from build123d import *

# Parameters (mm, degrees)
SKETCH1_W               = 12.7
SKETCH1_H               = 19.05
BOSS_EXTRUDE1_DEPTH     = 152.4
SKETCH2_R               = 4.5640625
CUT_EXTRUDE1_DEPTH      = 1
CUT_EXTRUDE1_DEPTH_BACK = 13.7
SKETCH6_R               = 2.778125
CUT_EXTRUDE4_DEPTH      = 1
CUT_EXTRUDE4_DEPTH_BACK = 20.05


with BuildPart() as part:
    # Sketch1 → Boss-Extrude1 (new body, symmetric)
    with BuildSketch(Plane(origin=(0, 0, 0), x_dir=(0, 0, -1), z_dir=(1, 0, 0))):
        Rectangle(SKETCH1_W, SKETCH1_H)
    extrude(amount=BOSS_EXTRUDE1_DEPTH, both=True)

    # Sketch2 → Cut-Extrude1 (cut, two sides)
    with BuildSketch(Plane.XY.offset(6.35)) as cut_extrude1_sk:
        with Locations((139.7, 1.905)):
            Circle(SKETCH2_R)
        with Locations((-139.7, 1.905)):
            Circle(SKETCH2_R)
    extrude(amount=CUT_EXTRUDE1_DEPTH, mode=Mode.SUBTRACT)
    extrude(cut_extrude1_sk.sketch, amount=-CUT_EXTRUDE1_DEPTH_BACK, mode=Mode.SUBTRACT)

    # Sketch6 → Cut-Extrude4 (cut, two sides)
    with BuildSketch(Plane(origin=(0, 9.525, 0), x_dir=(1, 0, 0), z_dir=(0, 1, 0))) as cut_extrude4_sk:
        with Locations((-127, 0)):
            Circle(SKETCH6_R)
        with Locations((127, 0)):
            Circle(SKETCH6_R)
    extrude(amount=CUT_EXTRUDE4_DEPTH, mode=Mode.SUBTRACT)
    extrude(cut_extrude4_sk.sketch, amount=-CUT_EXTRUDE4_DEPTH_BACK, mode=Mode.SUBTRACT)


solid = part.part
The listing builds one solid part. Answer for the finished solid, in the listing's coordinates (mm). Give positions to 0.01 mm unless a question says otherwise; leave off trailing zeros. Loops run counter-clockwise (first coordinate to the right, second up) from the corner with the lowest first, then second, coordinate; pieces in that order, holes last.
Item 1: Determine the mould class of faces 1 (the flat face through (152.4, 0, 0)), 2 (the flat face through (2, 0, -6.35)), 3 (the cylindrical face through (-144.26, 2.11, 0.09)) for opening direction X: +X half, -X half, draft (parallel to the pull), parting line (faces both ways), or undercut.
Derived:
face 1: +X half
face 2: draft
face 3: undercut
Item 2: A cutting plane is placed at B-B (z = 0). Give the vertices of the cut face in (x, y) (3 decimals), then the cut area to 3 significant figures.
Derived:
outline: (-152.4, -9.525) - (-129.778, -9.525) - (-129.778, 9.525) - (-152.4, 9.525) - close; (-124.222, -9.525) - (124.222, -9.525) - (124.222, 9.525) - (-124.222, 9.525) - close; (129.778, -9.525) - (152.4, -9.525) - (152.4, 9.525) - (129.778, 9.525) - close; hole circle Ø9.128 at (-139.7, 1.905); hole circle Ø9.128 at (139.7, 1.905)
area: 5,460 mm2
Item 3: Find the intervals of material crossed by line 1 along X through (y, z) = (-5, -0.5); line 2 along Y through (x, z) = (-139.7, 2.5) (3 decimals); line 3 along Z through (x, y) = (-127, 5.5), in increasing order.
Derived:
line 1: x = -152.4 to -129.73, -124.27 to 124.27, 129.73 to 152.4
line 2: y = -9.525 to -2.659, 6.469 to 9.525
line 3: z = -6.35 to -2.78, 2.78 to 6.35
Item 4: A cutting plane is placed at A-A (x = -139.7). Give the vertices of the cut face in (y, z) (3 decimals), then the cut area to 3 significant figures.
Derived:
outline: (-9.525, -6.35) - (-2.659, -6.35) - (-2.659, 6.35) - (-9.525, 6.35) - close; (6.469, -6.35) - (9.525, -6.35) - (9.525, 6.35) - (6.469, 6.35) - close
area: 126 mm2
Item 5: A cutting plane is placed at C-C (x = 127). Give the vertices of the cut face in (y, z) (3 decimals).
Derived:
outline: (-9.525, -6.35) - (9.525, -6.35) - (9.525, -2.778) - (-9.525, -2.778) - close; (-9.525, 2.778) - (9.525, 2.778) - (9.525, 6.35) - (-9.525, 6.35) - close
